```python
from build123d import *

# Parameters (mm, degrees)
SKETCH_3_R          = 32.5
CUT_EXTRUDE_1_DEPTH = 4
MM_1_D              = 8
MM_1_DEPTH          = 15
MM_1_TIP            = 2.403442476
CUT_EXTRUDE_2_REACH = 72.089
SKETCH_6_R          = 3
CHAMFER_1_SIZE      = 0.5


with BuildPart() as part:
    # 草图1 → 旋转1 (revolve)
    with BuildSketch(Plane(origin=(0, 0, 0), x_dir=(0, 0, -1), z_dir=(1, 0, 0)), mode=Mode.PRIVATE) as revolve_1_sk:
        Polygon((0, 0), (0, 47.5), (11, 47.5), (11, 19), (12, 19), (12, 15), (31, 15), (31, 0), align=None)
    revolve(revolve_1_sk.sketch.rotate(Axis((0, 0, 0), (0, 0, 1)), 90), axis=Axis((0, 0, 0), (0, 0, 1)))

    # 草图3 → 切除-拉伸1 (cut)
    with BuildSketch(Plane.XY):
        Circle(SKETCH_3_R)
    extrude(amount=-CUT_EXTRUDE_1_DEPTH, mode=Mode.SUBTRACT)

    # 大小mm 暗销孔1
    with Locations(Plane(origin=(0, 0, -31), x_dir=(-1, 0, 0), z_dir=(0, 0, -1))):
        with Locations((0, 0)):
            Hole(MM_1_D / 2, depth=MM_1_DEPTH)
            with Locations((0, 0, -(MM_1_DEPTH + MM_1_TIP / 2))):  # 118° drill point
                Cone(0, MM_1_D / 2, MM_1_TIP, mode=Mode.SUBTRACT)

    # 草图6 → 切除-拉伸2 (cut, up to next)
    with BuildSketch(Plane(origin=(0, 0, -11), x_dir=(-1, 0, 0), z_dir=(0, 0, -1)), mode=Mode.PRIVATE) as cut_extrude_2_sk1:
        with Locations((0, 40)):
            Circle(SKETCH_6_R)
    cut_extrude_2_tool1 = extrude(cut_extrude_2_sk1.sketch, amount=-CUT_EXTRUDE_2_REACH, mode=Mode.PRIVATE) & part.part
    # 草图6 → 切除-拉伸2 (cut, up to next)
    with BuildSketch(Plane(origin=(0, 0, -11), x_dir=(-1, 0, 0), z_dir=(0, 0, -1)), mode=Mode.PRIVATE) as cut_extrude_2_sk2:
        with Locations((28.284271247, 28.284271247)):
            Circle(SKETCH_6_R)
    cut_extrude_2_tool2 = extrude(cut_extrude_2_sk2.sketch, amount=-CUT_EXTRUDE_2_REACH, mode=Mode.PRIVATE) & part.part
    # 草图6 → 切除-拉伸2 (cut, up to next)
    with BuildSketch(Plane(origin=(0, 0, -11), x_dir=(-1, 0, 0), z_dir=(0, 0, -1)), mode=Mode.PRIVATE) as cut_extrude_2_sk3:
        with Locations((40, 0)):
            Circle(SKETCH_6_R)
    cut_extrude_2_tool3 = extrude(cut_extrude_2_sk3.sketch, amount=-CUT_EXTRUDE_2_REACH, mode=Mode.PRIVATE) & part.part
    # 草图6 → 切除-拉伸2 (cut, up to next)
    with BuildSketch(Plane(origin=(0, 0, -11), x_dir=(-1, 0, 0), z_dir=(0, 0, -1)), mode=Mode.PRIVATE) as cut_extrude_2_sk4:
        with Locations((28.284271247, -28.284271247)):
            Circle(SKETCH_6_R)
    cut_extrude_2_tool4 = extrude(cut_extrude_2_sk4.sketch, amount=-CUT_EXTRUDE_2_REACH, mode=Mode.PRIVATE) & part.part
    # 草图6 → 切除-拉伸2 (cut, up to next)
    with BuildSketch(Plane(origin=(0, 0, -11), x_dir=(-1, 0, 0), z_dir=(0, 0, -1)), mode=Mode.PRIVATE) as cut_extrude_2_sk5:
        with Locations((0, -40)):
            Circle(SKETCH_6_R)
    cut_extrude_2_tool5 = extrude(cut_extrude_2_sk5.sketch, amount=-CUT_EXTRUDE_2_REACH, mode=Mode.PRIVATE) & part.part
    # 草图6 → 切除-拉伸2 (cut, up to next)
    with BuildSketch(Plane(origin=(0, 0, -11), x_dir=(-1, 0, 0), z_dir=(0, 0, -1)), mode=Mode.PRIVATE) as cut_extrude_2_sk6:
        with Locations((-28.284271247, -28.284271247)):
            Circle(SKETCH_6_R)
    cut_extrude_2_tool6 = extrude(cut_extrude_2_sk6.sketch, amount=-CUT_EXTRUDE_2_REACH, mode=Mode.PRIVATE) & part.part
    # 草图6 → 切除-拉伸2 (cut, up to next)
    with BuildSketch(Plane(origin=(0, 0, -11), x_dir=(-1, 0, 0), z_dir=(0, 0, -1)), mode=Mode.PRIVATE) as cut_extrude_2_sk7:
        with Locations((-40, 0)):
            Circle(SKETCH_6_R)
    cut_extrude_2_tool7 = extrude(cut_extrude_2_sk7.sketch, amount=-CUT_EXTRUDE_2_REACH, mode=Mode.PRIVATE) & part.part
    # 草图6 → 切除-拉伸2 (cut, up to next)
    with BuildSketch(Plane(origin=(0, 0, -11), x_dir=(-1, 0, 0), z_dir=(0, 0, -1)), mode=Mode.PRIVATE) as cut_extrude_2_sk8:
        with Locations((-28.284271247, 28.284271247)):
            Circle(SKETCH_6_R)
    cut_extrude_2_tool8 = extrude(cut_extrude_2_sk8.sketch, amount=-CUT_EXTRUDE_2_REACH, mode=Mode.PRIVATE) & part.part
    add(cut_extrude_2_tool1.solids().sort_by_distance((0, 40, -11))[0], mode=Mode.SUBTRACT)
    add(cut_extrude_2_tool2.solids().sort_by_distance((-28.284271, 28.284271, -11))[0], mode=Mode.SUBTRACT)
    add(cut_extrude_2_tool3.solids().sort_by_distance((-40, 0, -11))[0], mode=Mode.SUBTRACT)
    add(cut_extrude_2_tool4.solids().sort_by_distance((-28.284271, -28.284271, -11))[0], mode=Mode.SUBTRACT)
    add(cut_extrude_2_tool5.solids().sort_by_distance((0, -40, -11))[0], mode=Mode.SUBTRACT)
    add(cut_extrude_2_tool6.solids().sort_by_distance((28.284271, -28.284271, -11))[0], mode=Mode.SUBTRACT)
    add(cut_extrude_2_tool7.solids().sort_by_distance((40, 0, -11))[0], mode=Mode.SUBTRACT)
    add(cut_extrude_2_tool8.solids().sort_by_distance((28.284271, 28.284271, -11))[0], mode=Mode.SUBTRACT)

    # 倒角1
    chamfer_1_edges = [part.edges().sort_by_distance(p)[0] for p in [
        (-4, 0, -31),
        (15, 0, -31),
        (47.5, 0, -11),
        (47.5, 0, 0),
    ]]
    chamfer(chamfer_1_edges, length=CHAMFER_1_SIZE)


solid = part.part
```
The listing builds one solid part. Answer for the finished solid, in the listing's coordinates (mm). A direction names the side the tool comes from. Coordinates: 2 decimals unless noted, no trailing zeros. Loops run counter-clockwise (first coordinate to the right, second up) from the corner with the lowest first, then second, coordinate; pieces in that order, holes last. Notation, with made-up numbers: M 78.25,64.5 L 106.25,64.5 A28 ccw 106.25,97.5 Z; hole C 8.25,83 d5. An arc over 180 degrees is marked long. Answer as a JSON object with one key per item and string values. Group by question number.
Item 1: Section B-B (z = -9) is taken. Give the number of separate pieces and of enclosed holes in the cut face, and give its area (3 significant figures).
Item 2: Which of the six approach directions +Z, -Z, +X, -X, +Y, -Y give full straight-line access (tool end or side, diameter ignored) to faces 1 (the face through (-31.056, 27.135, -5.577)), 2 (the face through (0, 0, -4)), 3 (the face through (4.119, 18.548, -11.507))?
Item 3: Section A-A (z = -24.5) is taken. Write down the section's boundary in (x, y), and give its area (3 significant figures).
Item 4: Each of these flat-tipped pins is pushed along its axis until it touches: P1, Ø12, axis at y = -18.5, z = -14.5, coming from the -X side; P2, Ø6.5, axis at x = 0, y = 0, coming from the -Z side; P3, Ø8, axis at x = 28.28, y = 28.28, coming from the -Z side; P4, Ø9.5, axis at x = -28.28, y = -28.28, coming from the +Z side. Where does it stop, or does it pass through?
Item 5: Consider L1, parallel to Y at x = 0, z = -3.5; L2, parallel to Y at x = 0, z = -6.75; L3, parallel to Y at x = 0, z = -26. Determine where each line is inside the solid, lowest interval first.
Item 6: Determine the mould class of faces 4 (the face through (3.4, -3.4, -31)), 5 (the face through (10.3, 46.37, -5.57)), 6 (the face through (-31.056, -29.433, -5.577)) for opening direction X: +X half, -X half, draft (parallel to the pull), parting line (faces both ways), or undercut.
Solved:
{
 "1": {"separate pieces": "1", "enclosed holes": "8", "area": "6,860 mm2"},
 "2": {"face 1": "+Z, -Z", "face 2": "+Z", "face 3": "-Z"},
 "3": {"outline": "C 0,0 d30; hole C 0,0 d8", "area": "657 mm2"},
 "4": {"P1": "stops at x = -45.38", "P2": "stops at z = -15.55", "P3": "stops at z = -11", "P4": "stops at z = 0"},
 "5": {"L1": "y = -47.5 to -43, -37 to -32.5, 32.5 to 37, 43 to 47.5", "L2": "y = -47.5 to -43, -37 to 37, 43 to 47.5", "L3": "y = -15 to -4, 4 to 15"},
 "6": {"face 4": "draft", "face 5": "parting line", "face 6": "undercut"}
}
